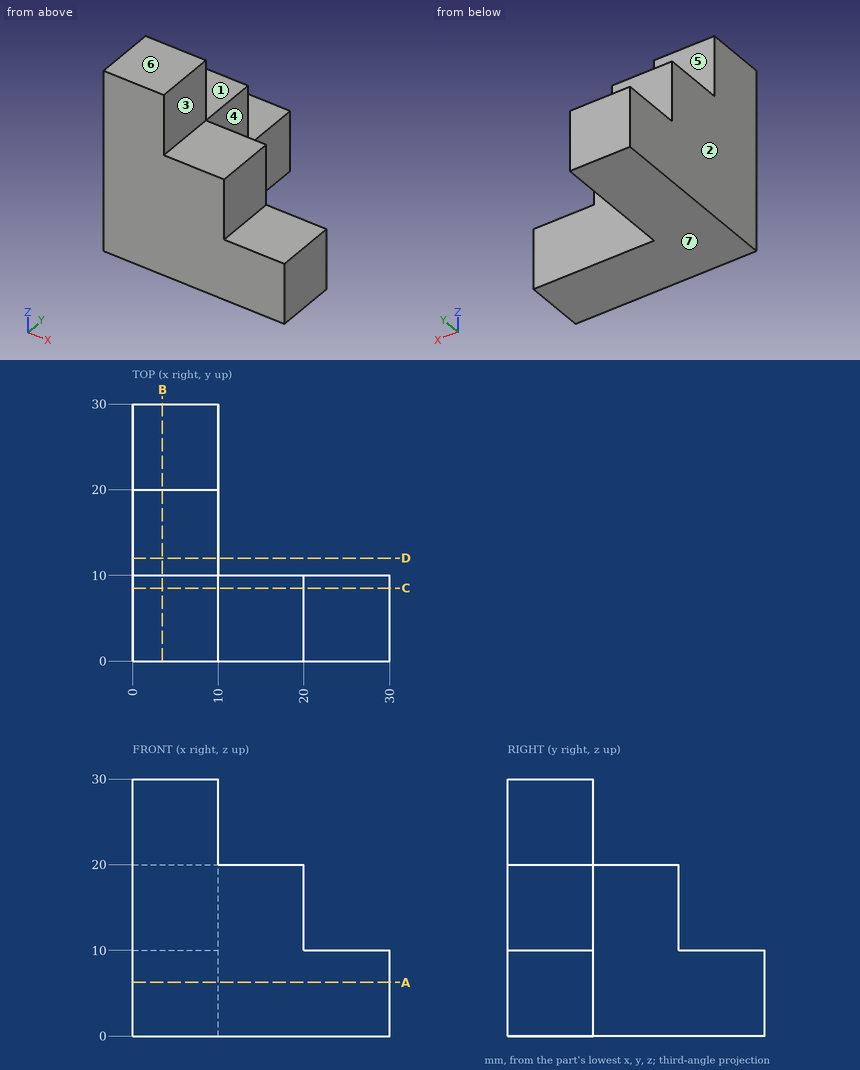
Input: dimensioned drawing with shaded views. Units: mm. Origin: part minimum x, y, z. A direction names the side the tool comes from. Coordinates: 2 decimals unless noted, no trailing zeros. Loops run counter-clockwise (first coordinate to the right, second up) from the corner with the lowest first, then second, coordinate; pieces in that order, holes last. Notation, with made-up numbers: (26, 36.5) -> (37, 36.5) arc R32 ccw to (37, 65.5) -> close; hole circle Ø6 at (49, -5). An arc over 180 degrees is marked (long way). Use a Markdown table: item, result. Add a question column.
(1) Pin query (flat end, axial travel): pin 1 Ø10 at (x, z) = (25, 8.5) entering from +Y; pin 2 Ø16 at (y, z) = (23.5, 14) entering from +X; pin 3 Ø5 at (x, y) = (5.5, 16.5) entering from +Z. Return the tip coordinate at first contact, or that it passes through.
(2) Mould query, pull axis Z, two halves, no side actions, for the marked faces 5, 6 and 7. Classes: pulls with the +Z half, pulls with the -Z half, needs draft (parallel to the pull), parting line crosses it, or undercut.
(3) Section query A-A, the plane z = 6.25. Return loops of the section in (x, y), plus the area to 3 significant figures.
(4) Access query for the marked faces 1, 2, 3 and 4. Directions: +Z, -Z, +X, -X, +Y, -Y. A direction counts if a zero-diameter tool reaches every point of the face in a straight line with its end or side. Return the directions, or none.
(5) Line query: line 1 along X through (y, z) = (6.5, 25). Output: solid intervals per line, ascending.
(6) Section query D-D, the plane y = 12. Return loops of the section in (x, z), plus the area to 3 significant figures.
(7) Section query B-B, the plane x = 3.5. Return loops of the section in (y, z).
Answer:
| question | item | result |
|---|---|---|
| 1 | pin 1 | stops at y = 10 |
| 1 | pin 2 | stops at x = 10 |
| 1 | pin 3 | stops at z = 20 |
| 2 | face 5 | needs draft |
| 2 | face 6 | pulls with the +Z half |
| 2 | face 7 | pulls with the -Z half |
| 3 | outline | (0, 0) -> (30, 0) -> (30, 10) -> (10, 10) -> (10, 30) -> (0, 30) -> close |
| 3 | area | 500 mm^2 |
| 4 | face 1 | +Z, +X, -X, +Y |
| 4 | face 2 | +Z, -Z, -X, +Y, -Y |
| 4 | face 3 | +Z, +X, +Y, -Y |
| 4 | face 4 | +Z, -Z, +X, +Y |
| 5 | line 1 | x = 0 to 10 |
| 6 | outline | (0, 0) -> (10, 0) -> (10, 20) -> (0, 20) -> close |
| 6 | area | 200 mm^2 |
| 7 | outline | (0, 0) -> (30, 0) -> (30, 10) -> (20, 10) -> (20, 20) -> (10, 20) -> (10, 30) -> (0, 30) -> close |
